from build123d import *

# Parameters (mm, degrees)
F2_R     = 5
F3_DEPTH = 10
F4_R     = 1.75
F5_DEPTH = 25


with BuildPart() as f1:
    # F0 (on Top) → F1 (revolve)
    with BuildSketch(Plane.XY):
        Polygon((2.124551, 4), (2.124551, 0), (34.324551, 0), (34.324551, 2), (33.824551, 2), (33.824551, 10), (34.324551, 10), (34.324551, 12), (26.324551, 12), (26.324551, 4), align=None)
    revolve(axis=Axis((2.124551, 2, 0), (0, -1, 0)))

    # F2 (on face) → F3 (join)
    with BuildSketch(Plane(origin=(0, 4, 0), x_dir=(-1, 0, 0), z_dir=(0, 1, 0))):
        with Locations((-2.124551, 0)):
            Circle(F2_R)
    extrude(amount=F3_DEPTH)

    # F4 (on face) → F5 (cut)
    with BuildSketch(Plane(origin=(0, 14, 0), x_dir=(-1, 0, 0), z_dir=(0, 1, 0))):
        with Locations((-2.124551, 0)):
            Circle(F4_R)
    extrude(amount=-F5_DEPTH, mode=Mode.SUBTRACT)


solid = f1.part
Can you work these out from the model? Positions are in its coordinate system, mm. A direction names the side the tool comes from. Round coordinates to 2 decimals unless told otherwise and drop trailing zeros. Write each loop counter-clockwise with the first axis right and the second up, starting at its lowest first coordinate (ties: lowest second). Pieces come first, ordered by that corner, then holes. Notation, with made-up numbers: M 3.5,9.5 L 49.5,9.5 A15 ccw 49.5,13.5 Z; hole C 9,89.5 d4. An arc over 180 degrees is marked long. Use a Markdown table: item, result.
Item 1: I want a section at B-B (y = 6.5). List the corners of the cut face in (x, z) for me, and give its area (3 significant figures).
Found:
| item | result |
|---|---|
| outline | C 2.12,0 d63.4; C 2.12,0 d10; hole C 2.12,0 d48.4; hole C 2.12,0 d3.5 |
| area | 1,390 mm2 |
Item 2: I want a section at D-D (x = 16). List the corners of the cut face in (y, z) for me.
Found:
| item | result |
|---|---|
| outline | M 0,-29.06 L 2,-29.06 L 2,-28.5 L 10,-28.5 L 10,-29.06 L 12,-29.06 L 12,-19.83 L 4,-19.83 L 4,19.83 L 12,19.83 L 12,29.06 L 10,29.06 L 10,28.5 L 2,28.5 L 2,29.06 L 0,29.06 Z |
Item 3: I want a section at A-A (z = 0). List the corners of the cut face in (x, y) for me, and give its area (3 significant figures).
Found:
| item | result |
|---|---|
| outline | M -30.08,0 L 0.37,0 L 0.37,14 L -2.88,14 L -2.88,4 L -22.08,4 L -22.08,12 L -30.08,12 L -30.08,10 L -29.58,10 L -29.58,2 L -30.08,2 Z; M 3.87,0 L 34.32,0 L 34.32,2 L 33.82,2 L 33.82,10 L 34.32,10 L 34.32,12 L 26.32,12 L 26.32,4 L 7.12,4 L 7.12,14 L 3.87,14 Z |
| area | 429 mm2 |
Item 4: If I drill on line 1 along Z through (x, y) = (-9.5, 6.5); line 2 along Y through (x, z) = (-9, -8); line 3 along Z through (x, y) = (15.5, 7), over which ranges is the centre line in solid material (lowest first)? Write a range as [from, to].
Found:
| item | result |
|---|---|
| line 1 | z = [-29.49, -21.23], [21.23, 29.49] |
| line 2 | y = [0, 4] |
| line 3 | z = [-28.74, -20.17], [20.17, 28.74] |
Item 5: Which directions (+Z, -Z, +X, -X, +Y, -Y) give clear straight access to the entire face, cutting with the end or side of a thin tool? Please do faces 4 (the face through (-22, 10, -21)), 5 (the face through (-2.645, 8.93, 1.502)), 6 (the face through (-23.43, 1.01, -19.59)).
Found:
| item | result |
|---|---|
| face 4 | none |
| face 5 | +Y |
| face 6 | +Y, -Y |
Item 6: I want a section at C-C (x = 3). List the corners of the cut face in (y, z) for me.
Found:
| item | result |
|---|---|
| outline | M 0,-32.19 L 2,-32.19 L 2,-31.69 L 10,-31.69 L 10,-32.19 L 12,-32.19 L 12,-24.18 L 4,-24.18 L 4,-4.92 L 14,-4.92 L 14,-1.52 L 0,-1.52 Z; M 0,1.52 L 14,1.52 L 14,4.92 L 4,4.92 L 4,24.18 L 12,24.18 L 12,32.19 L 10,32.19 L 10,31.69 L 2,31.69 L 2,32.19 L 0,32.19 Z |
Item 7: For pin 1 Ø12 at (x, z) = (-23, 13) entering from +Y; pin 2 Ø2 at (x, z) = (1, -25) entering from -Y; pin 3 Ø1.5 at (y, z) = (9, 16.5) entering from +X; pin 4 Ø1.5 at (x, y) = (-5.5, 12.5) entering from +Z, each with a flat end and sliding along its axis, tell me the tip position at first contact or that it passes through.
Found:
| item | result |
|---|---|
| pin 1 | stops at y = 12 |
| pin 2 | stops at y = 0 |
| pin 3 | stops at x = 29.64 |
| pin 4 | stops at z = 31.42 |
Item 8: We'd pull the mould along Y, two halves only. Please class faces 1 (the face through (25.83, 2, -21.32)), 2 (the face through (3.513, 7.098, -1.065)), 3 (the face through (7, 12, 24)): released by +Y, released by -Y, zero draft, split by the parting line, or undercut.
Found:
| item | result |
|---|---|
| face 1 | undercut |
| face 2 | zero draft |
| face 3 | released by +Y |
